Verification items for the finished model (mm, model axes). A direction names the side the tool comes from. Round coordinates to 2 decimals unless told otherwise and drop trailing zeros. Write each loop counter-clockwise with the first axis right and the second up, starting at its lowest first coordinate (ties: lowest second). Pieces come first, ordered by that corner, then holes. Notation, with made-up numbers: (0, -15.5) - (24, -15.5) arc R25 ccw to (24, 5.5) - close; hole circle Ø3 at (-13, 59). An arc over 180 degrees is marked (long way). Answer as a JSON object with one key per item and string values.
```python
from build123d import *

# Parameters (mm, degrees)
SKETCH3_W                                         = 20
SKETCH3_H                                         = 60
SKETCH3_H_2                                       = 16.009607205
BOSS_EXTRUDE1_DEPTH                               = 50
SKETCH4_W                                         = 16.009607205
SKETCH4_H                                         = 30
CUT_EXTRUDE1_DEPTH                                = 10
FILLET4_R                                         = 15
CSK_FOR_8_FLAT_HEAD_MACHINE_SCREW_100_D           = 4.4958
CSK_FOR_8_FLAT_HEAD_MACHINE_SCREW_100_CSINK_D     = 8.4328
CSK_FOR_8_FLAT_HEAD_MACHINE_SCREW_100_CSINK_ANGLE = 100
SKETCH7_W                                         = 10
SKETCH7_H                                         = 20
CUT_EXTRUDE2_DEPTH                                = 50
SKETCH8_W                                         = 10
SKETCH8_H                                         = 20
CUT_EXTRUDE3_DEPTH                                = 13


with BuildPart() as part:
    # Sketch3 → Boss-Extrude1 (new body)
    with BuildSketch(Plane(origin=(0, 0, 0), x_dir=(1, 0, 0), z_dir=(0, 1, 0))):
        Rectangle(SKETCH3_W, SKETCH3_H)
        with Locations((20, 21.995196398)):
            Rectangle(SKETCH3_W, SKETCH3_H_2)
    extrude(amount=BOSS_EXTRUDE1_DEPTH)

    # Sketch4 → Cut-Extrude1 (cut)
    with BuildSketch(Plane(origin=(30, 0, 0), x_dir=(0, 0, -1), z_dir=(1, 0, 0))):
        with Locations((21.995196398, 25)):
            Rectangle(SKETCH4_W, SKETCH4_H)
    extrude(amount=-CUT_EXTRUDE1_DEPTH, mode=Mode.SUBTRACT)

    # Fillet4
    # the kernel refuses this fillet: 15 mm, written as the material it adds along each edge
    with BuildSketch(Plane(origin=(20, 10, -30), x_dir=(1, 0, 0), z_dir=(0, 0, 1))) as fillet4_piece_1:
        with BuildLine():
            CenterArc((15, 14.142135624), FILLET4_R, 180, 70.528779366)
            Line((0, 14.142135624), (-0.3, 14.142135624))
            Line((-0.3, 14.142135624), (-0.3, 0))
            Line((-0.3, 0), (0, -0.3))
            ThreePointArc((0, -0.3), (5, -0.3), (9.9, -0.282842712))
            Line((9.9, -0.282842712), (10, 0))
        make_face()
    extrude(amount=16.009607205)
    with BuildSketch(Plane(origin=(20, 40, -13.990392795), x_dir=(0, -1, 0), z_dir=(0, 0, -1))) as fillet4_piece_2:
        with BuildLine():
            CenterArc((14.142135624, -15), FILLET4_R, 90, 70.528779366)
            Line((0, -10), (-0.282842712, -9.9))
            ThreePointArc((-0.282842712, -9.9), (-0.3, -5), (-0.3, 0))
            Line((-0.3, 0), (0, 0.3))
            Line((0, 0.3), (14.142135624, 0.3))
            Line((14.142135624, 0.3), (14.142135624, 0))
        make_face()
    extrude(amount=16.009607205)

    # CSK for #8 Flat Head Machine Screw (100)1 (through all)
    with Locations(Plane.ZY.offset(10)):
        with Locations((23.5, 8), (23.5, 42)):
            CounterSinkHole(CSK_FOR_8_FLAT_HEAD_MACHINE_SCREW_100_D / 2, CSK_FOR_8_FLAT_HEAD_MACHINE_SCREW_100_CSINK_D / 2, counter_sink_angle=CSK_FOR_8_FLAT_HEAD_MACHINE_SCREW_100_CSINK_ANGLE)

    # Sketch7 → Cut-Extrude2 (cut)
    with BuildSketch(Plane(origin=(0, 0, -30), x_dir=(-1, 0, 0), z_dir=(0, 0, -1))):
        with Locations((2, 25)):
            Rectangle(SKETCH7_W, SKETCH7_H)
    extrude(amount=-CUT_EXTRUDE2_DEPTH, mode=Mode.SUBTRACT)

    # Sketch8 → Cut-Extrude3 (cut)
    with BuildSketch(Plane.ZY.offset(10)):
        with Locations((15, 25)):
            Rectangle(SKETCH8_W, SKETCH8_H)
    extrude(amount=-CUT_EXTRUDE3_DEPTH, mode=Mode.SUBTRACT)


solid = part.part
```
Q1. Material ranges on line 1 along Y through (x, z) = (6, 23.5); line 2 along X through (y, z) = (24, 8.5); line 3 along Y through (x, z) = (-1.5, 12), recorded low to high. Write a range as [from, to].
Geometry check:
{"line 1": "y = [0, 5.75], [10.25, 39.75], [44.25, 50]", "line 2": "x = [-10, -7], [3, 10]", "line 3": "y = [0, 15], [35, 50]"}
Q2. Release check for a two-part mould opening along Y. For faces 5 (the flat face through (10, 25, 8)), 6 (the flat face through (5, 50, -7)), 7 (the cylindrical face through (0.954, 43.519, 25.157)) record: released by +Y, released by -Y, zero draft, split by the parting line, or undercut.
Geometry check:
{"face 5": "zero draft", "face 6": "released by +Y", "face 7": "undercut"}
Q3. Section check D-D, the plane z = -4.5. Record the cut outline in (x, y).
Geometry check:
{"outline": "(-10, 0) - (10, 0) - (10, 50) - (-10, 50) - close; hole (-7, 15) - (3, 15) - (3, 35) - (-7, 35) - close"}
Q4. Gauge pin test, flat ends, axial feed: P1, Ø6, axis at x = 15, y = 19.5, coming from the +Z side; P2, Ø1.4, axis at y = 25.5, z = -21, coming from the +X side; P3, Ø4, axis at y = 39, z = 18, coming from the +X side. Record the tip position at first contact, or that the pin passes through.
Geometry check:
{"P1": "stops at z = -13.99", "P2": "stops at x = 20", "P3": "stops at x = 10"}
Q5. Section check C-C, the plane x = -1.5. Record the cut outline in (y, z), then the cut area to 3 significant figures.
Geometry check:
{"outline": "(0, -30) - (15, -30) - (15, 20) - (35, 20) - (35, -30) - (50, -30) - (50, 30) - (0, 30) - close; hole circle Ø4.5 at (8, 23.5); hole circle Ø4.5 at (42, 23.5)", "area": "1,970 mm2"}
Q6. Section check B-B, the plane y = 8. Record the cut outline in (x, z).
Geometry check:
{"outline": "(-10, -30) - (30, -30) - (30, -13.99) - (10, -13.99) - (10, 21.25) - (-8.35, 21.25) - (-10, 19.28) - close; (-10, 27.72) - (-8.35, 25.75) - (10, 25.75) - (10, 30) - (-10, 30) - close"}
Q7. Section check A-A, the plane z = 23.5. Record the cut outline in (x, y), then the cut area to 3 significant figures.
Geometry check:
{"outline": "(-10, 0) - (10, 0) - (10, 5.75) - (-8.35, 5.75) - (-10, 3.78) - close; (-10, 12.22) - (-8.35, 10.25) - (10, 10.25) - (10, 39.75) - (-8.35, 39.75) - (-10, 37.78) - close; (-10, 46.22) - (-8.35, 44.25) - (10, 44.25) - (10, 50) - (-10, 50) - close", "area": "814 mm2"}
Q8. Set-up check for faces 1 (the cylindrical face through (22.678, 15.588, -22.107)), 2 (the flat face through (18, 25, -13.99)), 3 (the flat face through (3, 25, -5)), 4 (the flat face through (-9, 25, 10)): record each of +Z, -Z, +X, -X, +Y, -Y from which the full face is reachable in a straight line by a thin tool's end or side.
Geometry check:
{"face 1": "+Z, -Z, +X", "face 2": "+Z, +X, +Y, -Y", "face 3": "-Z", "face 4": "-X"}
